Could you check a few things on this model? Use its own coordinates, in mm. Face numbers are marked on the shaded views. Round coordinates to 2 decimals unless told otherwise and drop trailing zeros. Loops run counter-clockwise (first coordinate to the right, second up) from the corner with the lowest first, then second, coordinate; pieces in that order, holes last. Notation, with made-up numbers: (-7, 5.25) - (16, 5.25) arc R19 ccw to (16, 41.25) - close; hole circle Ø10 at (-6, 71.25). An arc over 180 degrees is marked (long way). Answer as CSV lines item,"result". Start each with the question number.
1) We'd pull the mould along X, two halves only. Please class the marked faces 1, 2 and 3: pulls with the +X half, pulls with the -X half, needs draft (parallel to the pull), parting line crosses it, or undercut.
2) Suppose I cut it at C-C, the plane z = -0.35. Write out the boundary of the cut face in (x, y).
3) I'm going to push flat-ended pins straight in: pin 1 Ø1 at (y, z) = (3, 1) entering from -X; pin 2 Ø1.5 at (y, z) = (-2, 1) entering from +X. Where does each tip first touch, or does it pass through?
4) Suppose I cut it at A-A, the plane x = 0. Write out the boundary of the cut face in (y, z).
5) Please list where these lines run through material, in increasing order: line 1 along Y through (x, z) = (0, 0.75); line 2 along X through (y, z) = (-3, -0.9); line 3 along X through (y, z) = (-2, -0.15).
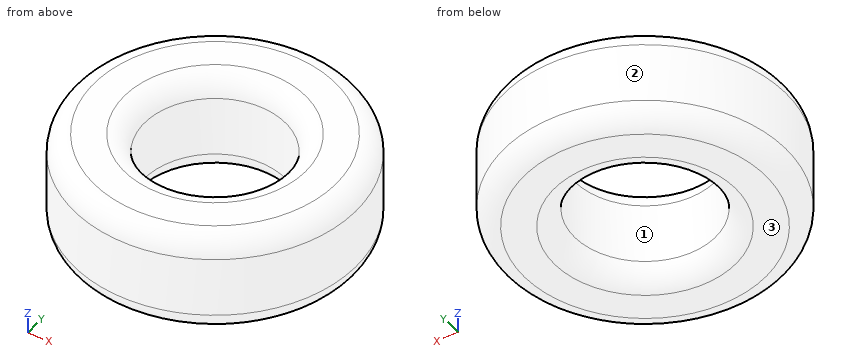
Autodesk Inventor part; units mm, degrees
sketch "Skizze1" plane through (0, 0, 0) normal (0, 0, 1) x (1, 0, 0)
  circle A0 centre (0, 0) radius 7
  circle A1 centre (0, 0) radius 3.5
  dimension "d0" = 14
  dimension "d1" = 7
extrude "Extrusion1" add sketch "Skizze1" along normal mid plane 5
fillet "Rundung1" radius 1 4 edges at (-7, 0, 2.5) (-7, 0, -2.5) (-3.5, 0, 2.5) (-3.5, 0, -2.5)
properties part number "KugelLager"
Filled sheet:
1,face 1,"undercut"
1,face 2,"parting line crosses it"
1,face 3,"needs draft"
2,outline,"circle Ø14 at (0, 0); hole circle Ø7 at (0, 0)"
3,pin 1,"x = -6.54"
3,pin 2,"x = 6.89"
4,outline,"(-7, -1.5) arc R1 ccw to (-6, -2.5) - (-4.5, -2.5) arc R1 ccw to (-3.5, -1.5) - (-3.5, 1.5) arc R1 ccw to (-4.5, 2.5) - (-6, 2.5) arc R1 ccw to (-7, 1.5) - close; (3.5, -1.5) arc R1 ccw to (4.5, -2.5) - (6, -2.5) arc R1 ccw to (7, -1.5) - (7, 1.5) arc R1 ccw to (6, 2.5) - (4.5, 2.5) arc R1 ccw to (3.5, 1.5) - close"
5,line 1,"-7 to -3.5, 3.5 to 7"
5,line 2,"-6.32 to -1.8, 1.8 to 6.32"
5,line 3,"-6.71 to -2.87, 2.87 to 6.71"
